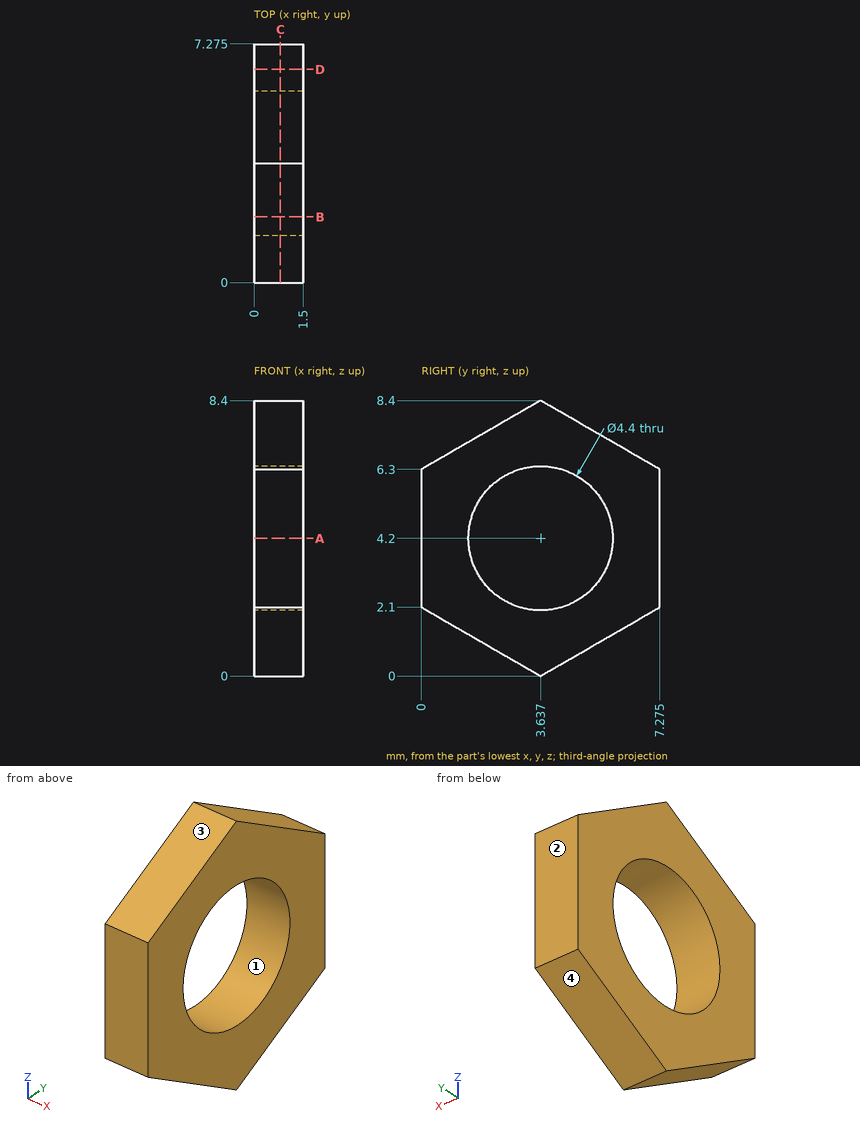
Can you work these out from the drawing? Everything is in mm from the part's minimum corner. Round coordinates to 2 decimals unless told otherwise and drop trailing zeros. Loops run counter-clockwise (first coordinate to the right, second up) from the corner with the lowest first, then second, coordinate; pieces in that order, holes last. Notation, with made-up numbers: (83, 38) - (108, 38) arc R15 ccw to (108, 57) - close; hole circle Ø1 at (36, 72.5). An arc over 180 degrees is marked (long way). Answer in a Markdown table with one row per item. Add a question column.
(1) I need wall thicknesses on line 1 along Z through (x, y) = (1.05, 4.25) (1 decimal); line 2 along Y through (x, z) = (1.3, 4.5) (1 decimal); line 3 along Y through (x, z) = (1.15, 5.5) (1 decimal). Which ranges of each line are inside material? Lowest first, please.
(2) If we section it at A-A (z = 4.2): Please give me the cut outline in (x, y) (1 decimal).
(3) If we mould it in two halves opening along Z, with no side actions, what happens to the marked faces 1, 2, 3 and 4? For each: pulls with the +Z half, pulls with the -Z half, needs draft (parallel to the pull), parting line crosses it, or undercut.
(4) If we section it at B-B (y = 2): Please give me the cut outline in (x, z) (1 decimal).
(5) If we section it at C-C (x = 0.8): Please give me the cut outline in (y, z) (1 decimal).
(6) If we section it at D-D (y = 6.5): Please give me the cut outline in (x, z).
Model answer:
| question | item | result |
|---|---|---|
| 1 | line 1 | z = 0.4 to 2.1, 6.3 to 8 |
| 1 | line 2 | y = 0 to 1.5, 5.8 to 7.3 |
| 1 | line 3 | y = 0 to 1.9, 5.4 to 7.3 |
| 2 | outline | (0, 0) - (1.5, 0) - (1.5, 1.4) - (0, 1.4) - close; (0, 5.8) - (1.5, 5.8) - (1.5, 7.3) - (0, 7.3) - close |
| 3 | face 1 | undercut |
| 3 | face 2 | needs draft |
| 3 | face 3 | pulls with the +Z half |
| 3 | face 4 | pulls with the -Z half |
| 4 | outline | (0, 0.9) - (1.5, 0.9) - (1.5, 2.7) - (0, 2.7) - close; (0, 5.7) - (1.5, 5.7) - (1.5, 7.5) - (0, 7.5) - close |
| 5 | outline | (0, 2.1) - (3.6, 0) - (7.3, 2.1) - (7.3, 6.3) - (3.6, 8.4) - (0, 6.3) - close; hole circle Ø4.4 at (3.6, 4.2) |
| 6 | outline | (0, 1.65) - (1.5, 1.65) - (1.5, 6.75) - (0, 6.75) - close |
